Autodesk Inventor part; units mm, degrees
ref_plane "YZ Plane" through (0, 0, 0) normal (1, 0, 0) x (0, 1, 0)
ref_plane "XZ Plane" through (0, 0, 0) normal (0, 1, 0) x (-1, 0, 0)
sketch "Skizze1" plane through (0, 0, 0) normal (0, 0, 1) x (1, 0, 0)
  circle A0 centre (0, 0) radius 2.5
  dimension "d0" = 5
extrude "Extrusion1" add sketch "Skizze1" along normal blind 6
sketch "Skizze3" plane through (0, 0, 0) normal (0, 1, 0) x (-1, 0, 0)
  line L0 (0, 24.65) -> (0, 24.65)
  line L1 (0, 24.65) -> (0, 5.15)
  line L2 (0, 5.15) -> (0, 5.15)
  line L3 (9.75, 14.9) -> (9.75, 14.9)
  arc A0 (9.75, 14.9) -> (0, 24.65) centre (0, 14.9) ccw
  arc A1 (0, 5.15) -> (9.75, 14.9) centre (0, 14.9) ccw
  line L4 (2.5, 6) -> (-2.5, 6)
  line L5 (2.5, 0) -> (-2.5, 0)
  line L6 (0, -5.3339) -> (0, 32.0031)
  point P0 (0, 0)
  point P1 (9.75, 24.65)
  point P2 (0, 14.9)
  point P3 (0, 24.65)
  dimension "d6" = 19.5
  dimension "d7" = 9.75
  dimension "d8" = 9.75
  dimension "d10" = 14.9
  dimension "d11" = 0
revolve "Umdrehung1" add sketch "Skizze3" angle 360 about axis through (0, 0, 24.65) along (0, 0, -1)
ref_plane "Arbeitsebene1" through (0, 0, 24.65) normal (0, 0, 1) x (1, 0, 0)
sketch "Skizze6" plane through (0, 0, 0) normal (0, 0, -1) x (-1, 0, 0)
  line L0 (-5, -5) -> (5, -5)
  line L1 (5, -5) -> (5, 5)
  line L2 (5, 5) -> (-5, 5)
  line L3 (-5, 5) -> (-5, -5)
  point P0 (0, 0)
  dimension "d21" = 5
  dimension "d22" = 5
  dimension "d23" = 10
  dimension "d24" = 5
extrude "Extrusion5" add sketch "Skizze6" along normal blind 7.6
fillet "Rundung6" radius 2 4 edges at (0, -5, 0) (-5, 0, 0) (5, 0, 0) (0, 5, 0)
fillet "Rundung7" radius 0.2 1 edges at (-2.5, 0, 0)
fillet "Rundung8" radius 0.2 8 edges at (-4.4142, -4.4142, -0.5858) (-5, -5, -4.8) (-4.4142, 4.4142, -0.5858) (-5, 5, -4.8) (4.4142, -4.4142, -0.5858) (5, -5, -4.8) (4.4142, 4.4142, -0.5858) (5, 5, -4.8)
sketch "Skizze7" plane through (0, 0, 24.65) normal (0, 0, 1) x (1, 0, 0)
  circle A0 centre (0, 0) radius 1.65
  dimension "d33" = 3.3
extrude "Extrusion6" cut sketch "Skizze7" against normal up to next
fillet "Rundung9" radius 0.2 2 edges at (0, -2.5, 5.476) (0, 2.5, 5.476)
sketch "Skizze8" plane through (0, 0, 24.65) normal (0, 0, 1) x (1, 0, 0)
  circle A0 centre (0, 0) radius 3.25
  dimension "d37" = 6.5
extrude "Extrusion7" cut sketch "Skizze8" against normal blind 15.4
properties part number "balljoint_male"
Build history of the part. All positions in model axes, mm. A direction names the side the tool comes from. Give positions to 0.01 mm unless a question says otherwise; leave off trailing zeros. Order: outer loops, then holes, each group sorted by start corner. A loop starts at its lowest first (then second) coordinate and runs counter-clockwise, first axis right, second up. Notation, with made-up numbers: M 21,44.25 L 30,44.25 A30 cw 30,81.25 Z; hole C -36.5,23.5 d7. An arc over 180 degrees is marked long. Put each result on its own line as item: value.
Item 1: Slice it at D-D, the plane z = 19. Write the cut outline in (x, y), plus the area to 3 significant figures.
From the geometry:
outline: C 0,0 d17.69; hole C 0,0 d6.5
area: 213 mm2
Item 2: 3-axis set-ups, long thin cutter, end or side, ignore diameter. For faces 1 (the flat face through (1.4, -1.4, 9.25)), 2 (the cylindrical face through (0.07, 4.43, -0.6)), 3 (the flat face through (5, 0, -5)): which of +Z, -Z, +X, -X, +Y, -Y reach the whole face in a straight line?
From the geometry:
face 1: +Z
face 2: +X, -X, +Y
face 3: -Z, +X, +Y, -Y
Item 3: Slice it at C-C, the plane y = 8. Write the cut outline in (x, z).
From the geometry:
outline: C 0,14.9 d11.15
Item 4: Two-plate mould, pull along Z, no slides. Class faces 4 (the flat face through (0, 2, -7.6)), 5 (the cylindrical face through (-2.579, -1.978, 16.775)), 6 (the cylindrical face through (-0.54, 2.44, 2.73)): +Z half, -Z half, draft (parallel to the pull), parting line (faces both ways), or undercut.
From the geometry:
face 4: -Z half
face 5: draft
face 6: undercut
Item 5: Slice it at B-B, the plane x = 6. Write the cut outline in (y, z).
From the geometry:
outline: C 0,14.9 d15.37
Item 6: Slice it at A-A, the plane z = -4.5. Write the cut outline in (x, y), plus the area to 3 significant figures.
From the geometry:
outline: M -5,-4.8 A0.2 ccw -4.8,-5 L 4.8,-5 A0.2 ccw 5,-4.8 L 5,4.8 A0.2 ccw 4.8,5 L -4.8,5 A0.2 ccw -5,4.8 Z; hole C 0,0 d3.3
area: 91.4 mm2
Item 7: Flat gauge pins, fed straight in: pin 1 Ø3 at (x, z) = (2, -4) entering from -Y; pin 2 Ø1.8 at (x, y) = (-1.5, 1) entering from +Z; pin 3 Ø1.5 at (y, z) = (-4, -4.5) entering from -X. Where does each tip first touch, or does it go through?
From the geometry:
pin 1: stops at y = -5
pin 2: stops at z = 9.25
pin 3: stops at x = -5
Item 8: Probe line 1 (Y direction, x = 0, z = -2); line 2 (X direction, y = 2, z = 16.5); line 3 (Y direction, x = 0, z = 3.75). List the from-to ranges inside material, lowest first. Write a range as [from, to].
From the geometry:
line 1: y = [-5, -1.65], [1.65, 5]
line 2: x = [-9.41, -2.56], [2.56, 9.41]
line 3: y = [-2.5, -1.65], [1.65, 2.5]
